The listing builds one solid part. Answer for the finished solid, in the listing's coordinates (mm). A direction names the side the tool comes from. Give positions to 0.01 mm unless a question says otherwise; leave off trailing zeros. Order: outer loops, then holes, each group sorted by start corner. A loop starts at its lowest first (then second) coordinate and runs counter-clockwise, first axis right, second up.
```python
from build123d import *

# Parameters (mm, degrees)
SKETCH2_W               = 5
SKETCH2_H               = 74.664160083
SKETCH2_W_2             = 10
SKETCH2_H_2             = 5
SKETCH2_R               = 1.15
BOSS_EXTRUDE1_DEPTH     = 1.5
SKETCH3_W               = 13
SKETCH3_H               = 74.664160083
BOSS_EXTRUDE2_DEPTH     = 1
SKETCH5_W               = 97.96
SKETCH5_H               = 74.648794292
BOSS_EXTRUDE3_DEPTH     = 1
SKETCH6_R               = 25
SKETCH6_R_2             = 23
BOSS_EXTRUDE4_DEPTH     = 17.5
SKETCH8_R               = 27.5
SKETCH8_R_2             = 23.5
BOSS_EXTRUDE6_DEPTH     = 2.5
SKETCH13_W              = 18
SKETCH13_H              = 23
BOSS_EXTRUDE7_DEPTH     = 1
SKETCH15_R              = 3.75
CUT_EXTRUDE3_DEPTH      = 1
BODY_MOVE_COPY2_ANGLE   = 90
SKETCH16_R              = 3.75
BOSS_EXTRUDE8_DEPTH     = 6
SKETCH17_R              = 0.9
CUT_EXTRUDE4_DEPTH      = 46
CUT_EXTRUDE4_DEPTH_BACK = 44


with BuildPart() as part:
    # Sketch2 → Boss-Extrude1 (new body)
    with BuildSketch(Plane.XY):
        with Locations((376.369557123, 140.674264472)):
            Rectangle(SKETCH2_W, SKETCH2_H)
        with Locations((368.869557123, 175.506344513)):
            Rectangle(SKETCH2_W_2, SKETCH2_H_2)
        with Locations((366.369557123, 175.506344513)):
            Circle(SKETCH2_R, mode=Mode.SUBTRACT)
        with Locations((368.869557123, 105.84218443)):
            Rectangle(SKETCH2_W_2, SKETCH2_H_2)
        with Locations((366.369557123, 105.84218443)):
            Circle(SKETCH2_R, mode=Mode.SUBTRACT)
    boss_extrude1 = extrude(amount=BOSS_EXTRUDE1_DEPTH)

    # Sketch3 → Boss-Extrude2 (add)
    with BuildSketch(Plane(origin=(378.869557123, 0, 0), x_dir=(0, 0, -1), z_dir=(1, 0, 0))):
        with Locations((5, 140.674264472)):
            Rectangle(SKETCH3_W, SKETCH3_H)
    extrude(amount=BOSS_EXTRUDE2_DEPTH)

    # Mirror3: Boss-Extrude1 across plane
    add(boss_extrude1.mirror(Plane(origin=(0, 0, -5), x_dir=(1, 0, 0), z_dir=(0, 0, -1))))


with BuildPart() as body_2:
    # Body-Move/Copy1: copy of part
    add(part.part.moved(Location((0, 0, 84.96))))


with BuildPart() as part_1:
    add(part.part)

    add(body_2.part)  # Boss-Extrude3 merges body 2
    # Sketch5 → Boss-Extrude3 (add)
    with BuildSketch(Plane(origin=(379.869557123, 0, 0), x_dir=(0, 0, -1), z_dir=(1, 0, 0))):
        with Locations((-37.48, 140.681947367)):
            Rectangle(SKETCH5_W, SKETCH5_H)
    extrude(amount=-BOSS_EXTRUDE3_DEPTH)

    # Sketch6 → Boss-Extrude4 (add)
    with BuildSketch(Plane.ZY.offset(-378.869557123)):
        with Locations(Location((37.48, 140.674264472, 0), (0, 0, 270))):
            Circle(SKETCH6_R)
        with Locations(Location((37.48, 140.674264472, 0), (0, 0, 270))):
            Circle(SKETCH6_R_2, mode=Mode.SUBTRACT)
    extrude(amount=BOSS_EXTRUDE4_DEPTH)

    # Sketch8 → Boss-Extrude6 (add)
    with BuildSketch(Plane.ZY.offset(-361.369557123)):
        with Locations(Location((37.48, 140.674264472, 0), (0, 0, 270))):
            Circle(SKETCH8_R)
        with Locations(Location((37.48, 140.674264472, 0), (0, 0, 270))):
            Circle(SKETCH8_R_2, mode=Mode.SUBTRACT)
    extrude(amount=BOSS_EXTRUDE6_DEPTH)

    # Sketch13 → Boss-Extrude7 (add)
    with BuildSketch(Plane.ZY.offset(-378.869557123)):
        with Locations((37.48, 189.506344513)):
            Rectangle(SKETCH13_W, SKETCH13_H)
        with Locations((37.48, 91.857550221)):
            Rectangle(SKETCH13_W, SKETCH13_H)
    extrude(amount=-BOSS_EXTRUDE7_DEPTH)

    # Sketch15 → Cut-Extrude3 (cut)
    with BuildSketch(Plane.ZY.offset(-378.869557123)):
        with Locations(Location((37.48, 195.006344513, 0), (0, 0, 270))):
            Circle(SKETCH15_R)
        with Locations(Location((37.48, 86.357550221, 0), (0, 0, 270))):
            Circle(SKETCH15_R)
    extrude(amount=-CUT_EXTRUDE3_DEPTH, mode=Mode.SUBTRACT)


with BuildPart() as part_2:
    # Body-Move/Copy2: moved
    add(part_1.part.rotate(Axis((371.869557123, 140.681947367, 0), (0, 0, 1)), BODY_MOVE_COPY2_ANGLE))

    # Sketch16 → Boss-Extrude8 (add)
    with BuildSketch(Plane(origin=(0, 148.681947367, 0), x_dir=(1, 0, 0), z_dir=(0, 1, 0))):
        Polygon((334.545159977, -28.48), (334.545159977, 11.5), (409.20932006, 11.5), (409.193954269, -28.48), (432.193954269, -28.48), (432.193954269, -46.48), (409.193954269, -46.48), (409.20932006, -86.46), (334.545159977, -86.46), (334.545159977, -46.48), (311.545159977, -46.48), (311.545159977, -28.48), align=None)
        with Locations((317.545159977, -37.48)):
            Circle(SKETCH16_R, mode=Mode.SUBTRACT)
        with Locations((426.193954269, -37.48)):
            Circle(SKETCH16_R, mode=Mode.SUBTRACT)
    extrude(amount=BOSS_EXTRUDE8_DEPTH)

    # Sketch17 → Cut-Extrude4 (cut, two sides)
    with BuildSketch(Plane.XY.offset(37.48)) as cut_extrude4_sk:
        with Locations(Location((371.877240018, 135.681947367, 0), (0, 0, 180))):
            Circle(SKETCH17_R)
    extrude(amount=CUT_EXTRUDE4_DEPTH, mode=Mode.SUBTRACT)
    extrude(cut_extrude4_sk.sketch, amount=-CUT_EXTRUDE4_DEPTH_BACK, mode=Mode.SUBTRACT)


solid = part_2.part
```
1) Find section A-A (y = 140.25). Count the separate pieces of the cut face and the enclosed holes in it, then the cut area to 3 significant figures.
Geometry says:
separate pieces: 9
enclosed holes: 1
area: 362 mm2
2) For a pull along Z with two mould halves and no side action, classify faces 1 (the flat face through (392, 127.682, 50)), 2 (the flat face through (323, 151, 46.48)), 3 (the flat face through (372, 144, 1.5)) as +Z half, -Z half, draft (parallel to the pull), parting line (faces both ways), or undercut.
Geometry says:
face 1: draft
face 2: +Z half
face 3: undercut
3) Straight lines are drawn through the part: probe 1 along Z at (x, y) = (371.5, 145.5); probe 2 along Z at (x, y) = (337.5, 144.5); probe 3 along Y at (x, z) = (367, -8). For each, find the intervals that lie inside material, in ascending order.
Geometry says:
probe 1: z = -11.5 to -10, 0 to 1.5, 12.48 to 14.48, 60.48 to 62.48, 73.46 to 74.96, 84.96 to 86.46
probe 2: z = -11.5 to -10, 0 to 1.5, 73.46 to 74.96, 84.96 to 86.46
probe 3: y = 147.68 to 154.68
4) Given P1, Ø3, axis at y = 133, z = 60, coming from the -X side; P2, Ø10, axis at x = 371, z = 51.5, coming from the -Y side; P3, Ø2.5, axis at x = 371.88, y = 135.68, coming from the +Z side, each flat-ended and moving along its own axis, determine where each tip first touches the part or whether it passes through.
Geometry says:
P1: stops at x = 358.34
P2: stops at y = 147.68
P3: stops at z = 62.48
5) Find section C-C (x = 402). Write down the section's boundary in (y, z), then the cut area to 3 significant figures.
Geometry says:
outline: (142.68, -11.5) - (154.68, -11.5) - (154.68, 86.46) - (142.68, 86.46) - (142.68, 84.96) - (147.68, 84.96) - (147.68, 74.96) - (142.68, 74.96) - (142.68, 73.46) - (147.68, 73.46) - (147.68, 1.5) - (142.68, 1.5) - (142.68, 0) - (147.68, 0) - (147.68, -10) - (142.68, -10) - close
area: 716 mm2
6) A tool of negligible diameter and unlimited length cuts with its end or side. For faces 4 (the cylindrical face through (393.123, 139.054, 28.671)), 5 (the cylindrical face through (346.9, 139.05, 38.58)), 6 (the flat face through (334.545, 150, 7)), 7 (the flat face through (371, 144, 73.46)), 8 (the flat face through (409.209, 142.4, -10.3)), from which of +Z, -Z, +X, -X, +Y, -Y can it reach the whole face along a straight path? Write none if from no direction.
Geometry says:
face 4: -Y
face 5: none
face 6: -Z, -X, +Y, -Y
face 7: +X, -X, -Y
face 8: -Z, +X, +Y, -Y
7) Find section B-B (z = 37.48). Write down the section's boundary in (x, y), then the cut area to 3 significant figures.
Geometry says:
outline: (311.55, 147.68) - (313.8, 147.68) - (313.8, 154.68) - (311.55, 154.68) - close; (321.3, 147.68) - (346.88, 147.68) - (346.88, 130.18) - (344.38, 130.18) - (344.38, 127.68) - (348.38, 127.68) - (348.38, 130.18) - (348.88, 130.18) - (348.88, 147.68) - (394.88, 147.68) - (394.88, 130.18) - (395.38, 130.18) - (395.38, 127.68) - (399.38, 127.68) - (399.38, 130.18) - (396.88, 130.18) - (396.88, 147.68) - (422.44, 147.68) - (422.44, 154.68) - (321.3, 154.68) - close; (429.94, 147.68) - (432.19, 147.68) - (432.19, 154.68) - (429.94, 154.68) - close
area: 830 mm2
